Geometry check sheet. Reference: drawing and pictorial views, mm from the part's lowest x, y, z. Give positions to 0.01 mm unless a question says otherwise; leave off trailing zeros. Write each loop counter-clockwise with the first axis right and the second up, starting at its lowest first coordinate (ties: lowest second). Pieces come first, ordered by that corner, then holes. Notation, with made-up numbers: (-21, 16) -> (24, 16) arc R16 cw to (24, 26) -> close; hole circle Ø3 at (-17, 71.25). An arc over 180 degrees is marked (long way). Return JSON: item names as keys, results as strings.
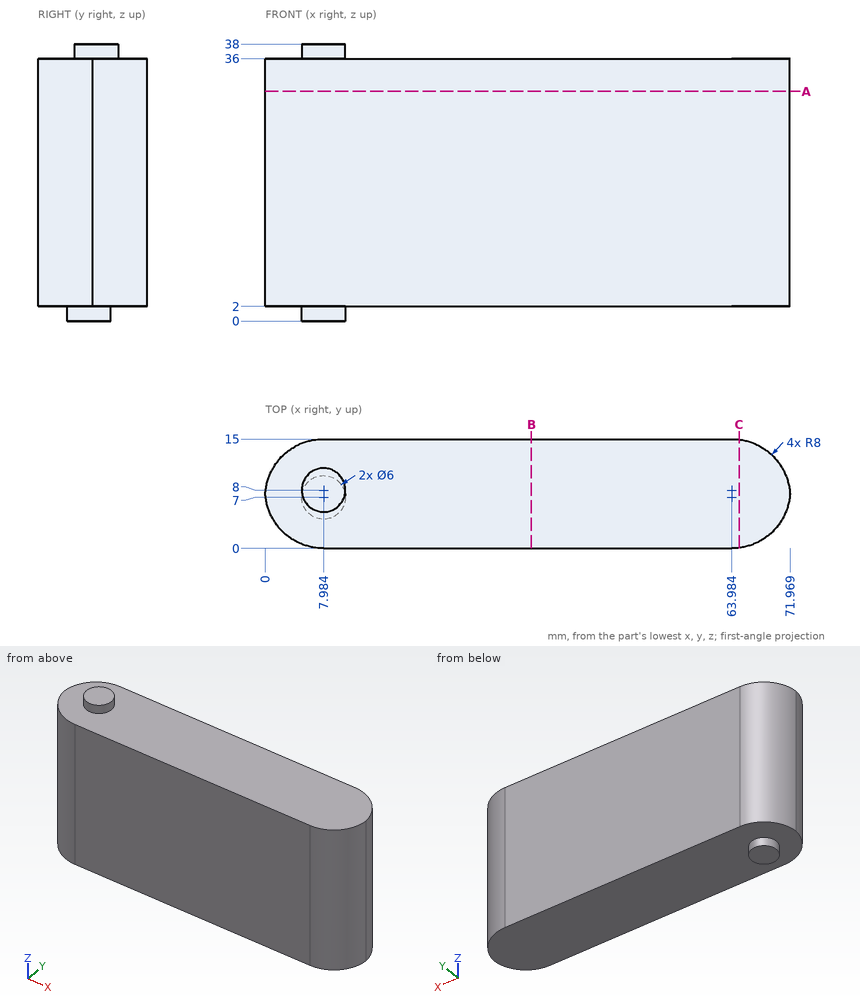
(1) Thickness scan on L1, parallel to Z at x = 37, y = 8; L2, parallel to Y at x = 64.5, z = 7.5; L3, parallel to X at y = 12, z = 22. Record the ranges inside material, lowest first.
Reply:
{"L1": "2 to 36", "L2": "0.02 to 14.98", "L3": "1.74 to 70.23"}
(2) Cross-section at A-A on z = 31.5. Enter the section's corners in (x, y) (1 decimal), then the cut area to 4 significant figures.
Reply:
{"outline": "(0, 7.5) arc R8 ccw to (8, 0) -> (64, 0) arc R8 ccw to (72, 7.5) arc R8 ccw to (64, 15) -> (8, 15) arc R8 ccw to start", "area": "1,025 mm^2"}
(3) Cross-section at C-C on x = 65. Enter the section's corners in (y, z) (1 decimal).
Reply:
{"outline": "(0.1, 2) -> (14.9, 2) -> (14.9, 36) -> (0.1, 36) -> close"}
(4) Depth check by flat-ended pin: pin 1 Ø2 at (y, z) = (9.5, 29.5) entering from +X; pin 2 Ø4 at (x, y) = (31.5, 2) entering from +Z; pin 3 Ø4.5 at (x, y) = (24.5, 7) entering from -Z. Enter the tip coordinate at first touch or a pass-through.
Reply:
{"pin 1": "x = 71.84", "pin 2": "z = 36", "pin 3": "z = 2"}
(5) Cross-section at B-B on x = 36.5. Enter the section's corners in (y, z), then the cut area to 3 significant figures.
Reply:
{"outline": "(0, 2) -> (15, 2) -> (15, 36) -> (0, 36) -> close", "area": "510 mm^2"}
